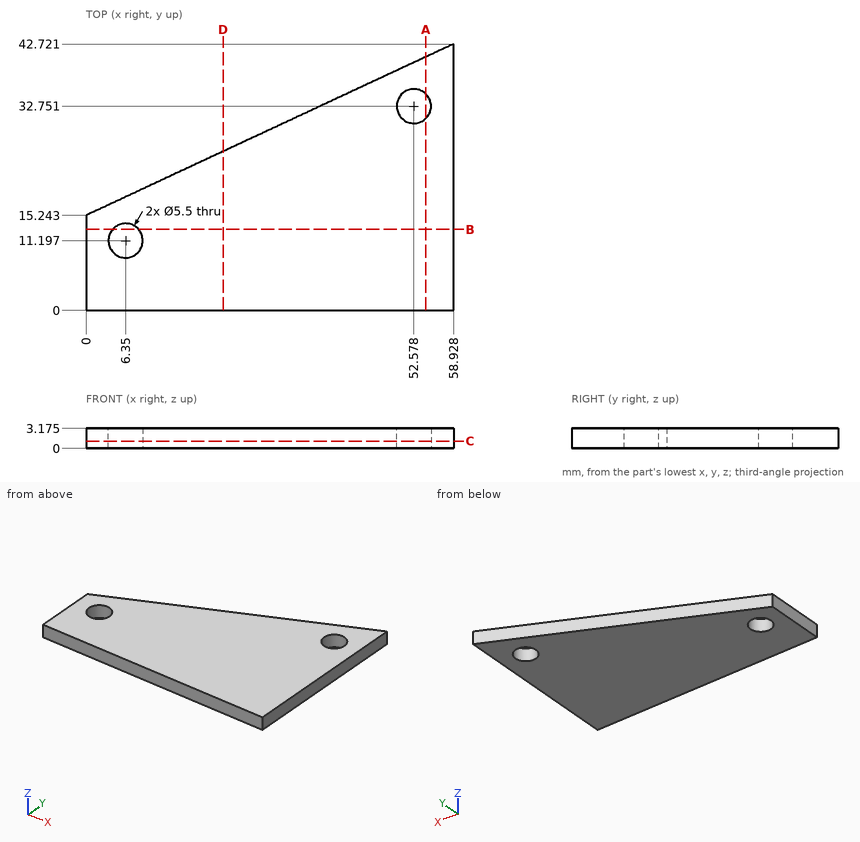
Print and shaded views of the part. All mm, measured from the part's lowest x, y and z. Round coordinates to 2 decimals unless told otherwise and drop trailing zeros. Write each loop counter-clockwise with the first axis right and the second up, starting at its lowest first coordinate (ties: lowest second). Pieces come first, ordered by that corner, then holes. Notation, with made-up numbers: (-33.75, -31) -> (2.25, -31) arc R23 ccw to (2.25, -13) -> close; hole circle Ø2 at (-9.5, 4). An arc over 180 degrees is marked (long way). Answer in a Markdown table with one row per item. Add a question column.
Item 1: Saw through at C-C, the plane z = 1.15. Write the cut outline in (x, y).
Item 2: Saw through at B-B, the plane y = 13. Write the cut outline in (x, z) (1 decimal), then the cut area to 3 significant figures.
Item 3: Drill centre lines: line 1 (Y direction, x = 6.35, z = 1.1) (1 decimal); line 2 (X direction, y = 32.5, z = 1.5) (1 decimal); line 3 (Y direction, x = 6, z = 0.2) (1 decimal). Where is each one in solid material? Low to high. Write a range as from..to.
Item 4: Drop a flat-ended pin along its axis: pin 1 Ø1.5 at (x, z) = (9.5, 0.5) entering from -Y. Give the stop position or say it passes through.
Item 5: Saw through at A-A, the plane x = 54.5. Write the cut outline in (y, z) (1 decimal), then the cut area to 3 significant figures.
Item 6: Saw through at D-D, the plane x = 22. Write the cut outline in (y, z) (1 decimal).
Findings below:
| question | item | result |
|---|---|---|
| 1 | outline | (0, 0) -> (58.93, 0) -> (58.93, 42.72) -> (0, 15.24) -> close; hole circle Ø5.5 at (6.35, 11.2); hole circle Ø5.5 at (52.58, 32.75) |
| 2 | outline | (0, 0) -> (4.3, 0) -> (4.3, 3.2) -> (0, 3.2) -> close; (8.4, 0) -> (58.9, 0) -> (58.9, 3.2) -> (8.4, 3.2) -> close |
| 2 | area | 174 mm^2 |
| 3 | line 1 | y = 0..8.4, 13.9..18.2 |
| 3 | line 2 | x = 37..49.8, 55.3..58.9 |
| 3 | line 3 | y = 0..8.5, 13.9..18 |
| 4 | pin 1 | stops at y = 0 |
| 5 | outline | (0, 0) -> (30.8, 0) -> (30.8, 3.2) -> (0, 3.2) -> close; (34.7, 0) -> (40.7, 0) -> (40.7, 3.2) -> (34.7, 3.2) -> close |
| 5 | area | 117 mm^2 |
| 6 | outline | (0, 0) -> (25.5, 0) -> (25.5, 3.2) -> (0, 3.2) -> close |
